from build123d import *

# Parameters (mm, degrees)
F1_DEPTH     = 1016
F2_R         = 25.4
F3_T1_DEPTH  = 1143
F3_T4_ANGLE  = 90
F3_T6_ANGLE  = 90
F3_T8_ANGLE  = 90
F3_T10_ANGLE = 90
F4_T         = -2.54


# Not quite as in the source:
# - a fillet or chamfer that OpenCascade refuses, or shapes differently, is made with other operations: its cross-section is extruded or revolved along the edge and cut away or added


with BuildPart() as f1:
    # F0 (on Top) → F1 (new body)
    with BuildSketch(Plane.XY):
        Polygon((254, -254), (254, 0), (254, 254), (-254, 254), (-254, -254), align=None)
    extrude(amount=F1_DEPTH)

    # F2
    f2_edges = [f1.edges().sort_by_distance(p)[0] for p in [
        (-254, 0, 0),
        (0, 254, 0),
        (0, -254, 0),
        (254, 0, 0),
    ]]
    fillet(f2_edges, radius=F2_R)

    # F3: fillet of radius 50.8 on 4 edges, made by hand

    # F3_s2 → F3_t1 (cut)
    with BuildSketch(Plane.XY):
        with BuildLine():
            ThreePointArc((-203.2, 254), (-239.1210244843, 239.1210244843), (-254, 203.2))
            Line((-254, 203.2), (-254, 254))
            Line((-254, 254), (-203.2, 254))
        make_face()
        with BuildLine():
            ThreePointArc((-203.2, -254), (-239.1210244843, -239.1210244843), (-254, -203.2))
            Line((-254, -203.2), (-254, -254))
            Line((-254, -254), (-203.2, -254))
        make_face()
        with BuildLine():
            ThreePointArc((254, 203.2), (239.1210244843, 239.1210244843), (203.2, 254))
            Line((203.2, 254), (254, 254))
            Line((254, 254), (254, 203.2))
        make_face()
        with BuildLine():
            ThreePointArc((254, -203.2), (239.1210244843, -239.1210244843), (203.2, -254))
            Line((203.2, -254), (254, -254))
            Line((254, -254), (254, -203.2))
        make_face()
    extrude(amount=F3_T1_DEPTH, mode=Mode.SUBTRACT)

    # F3_s3 → F3_t4 (revolve, cut)
    with BuildSketch(Plane.XZ.offset(203.2)):
        with BuildLine():
            ThreePointArc((228.6, 0), (246.5605122421, 7.4394877579), (254, 25.4))
            Line((254, 25.4), (254, 0))
            Line((254, 0), (228.6, 0))
        make_face()
    revolve(axis=Axis((203.2, -203.2, 0), (0, 0, -1)), revolution_arc=F3_T4_ANGLE, mode=Mode.SUBTRACT)

    # F3_s5 → F3_t6 (revolve, cut)
    with BuildSketch(Plane.YZ.offset(203.2)):
        with BuildLine():
            ThreePointArc((228.6, 0), (246.5605122421, 7.4394877579), (254, 25.4))
            Line((254, 25.4), (254, 0))
            Line((254, 0), (228.6, 0))
        make_face()
    revolve(axis=Axis((203.2, 203.2, 0), (0, 0, -1)), revolution_arc=F3_T6_ANGLE, mode=Mode.SUBTRACT)

    # F3_s7 → F3_t8 (revolve, cut)
    with BuildSketch(Plane.YZ.offset(-203.2)):
        with BuildLine():
            ThreePointArc((-228.6, 0), (-246.5605122421, 7.4394877579), (-254, 25.4))
            Line((-254, 25.4), (-254, 0))
            Line((-254, 0), (-228.6, 0))
        make_face()
    revolve(axis=Axis((-203.2, -203.2, 0), (0, 0, -1)), revolution_arc=F3_T8_ANGLE, mode=Mode.SUBTRACT)

    # F3_s9 → F3_t10 (revolve, cut)
    with BuildSketch(Plane.XZ.offset(-203.2)):
        with BuildLine():
            ThreePointArc((-228.6, 0), (-246.5605122421, 7.4394877579), (-254, 25.4))
            Line((-254, 25.4), (-254, 0))
            Line((-254, 0), (-228.6, 0))
        make_face()
    revolve(axis=Axis((-203.2, 203.2, 0), (0, 0, -1)), revolution_arc=F3_T10_ANGLE, mode=Mode.SUBTRACT)

    # F4
    f4_openings = [f1.faces().sort_by_distance(p)[0] for p in [
        (0, 0, 1016),
    ]]
    offset(amount=F4_T, openings=f4_openings)


solid = f1.part
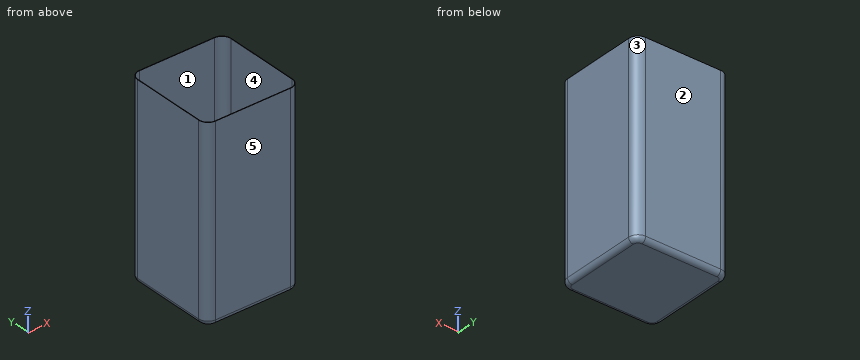
Design review of the part built by this model. Coordinates are the model's own, in mm. Face numbers are marked on the shaded views. A direction names the side the tool comes from. Coordinates: 2 decimals unless noted, no trailing zeros. Order: outer loops, then holes, each group sorted by start corner. A loop starts at its lowest first (then second) coordinate and runs counter-clockwise, first axis right, second up.
Item 1: The part is to be moulded in two halves that separate along X. For the marked faces 3, 4 and 5, say which applies: pulls with the +X half, pulls with the -X half, needs draft (parallel to the pull), parting line crosses it, or undercut.
Item 2: For pin 1 Ø1 at (x, y) = (34.5, -71.5) entering from +Z, flat-tipped, find the tip position at first contact; note if it passes through.
Item 3: Take a section at B-B, the plane x = 115.5. Write out the cut boundary in (y, z), then the cut area to 3 significant figures.
Item 4: For line 1 (X direction, y = -106, z = 292); line 2 (Z direction, x = -77, y = 9.5), list the stretches that pass through material, from the lowest coordinate up.
Item 5: For the marked faces 1 and 2, list the 3-axis set-ups (+Z, -Z, +X, -X, +Y, -Y) from which the entire face can be reached by the end or side of a thin tool; tool diameter is ignored.
Item 6: Take a section at A-A, the plane z = 389. Write out the cut boundary in (x, y).
The answers:
1. face 3: pulls with the +X half
1. face 4: undercut
1. face 5: needs draft
2. pin 1: stops at z = 2.54
3. outline: (-254, 25.4) arc R25.4 ccw to (-228.6, 0) - (228.6, 0) arc R25.4 ccw to (254, 25.4) - (254, 1016) - (251.46, 1016) - (251.46, 25.4) arc R22.86 cw to (228.6, 2.54) - (-228.6, 2.54) arc R22.86 cw to (-251.46, 25.4) - (-251.46, 1016) - (-254, 1016) - close
3. area: 6,390 mm2
4. line 1: x = -254 to -251.46, 251.46 to 254
4. line 2: z = 0 to 2.54
5. face 1: +Z
5. face 2: +Z, -Z, +X, -X, +Y
6. outline: (-254, -203.2) arc R50.8 ccw to (-203.2, -254) - (203.2, -254) arc R50.8 ccw to (254, -203.2) - (254, 203.2) arc R50.8 ccw to (203.2, 254) - (-203.2, 254) arc R50.8 ccw to (-254, 203.2) - close; hole (-251.46, -203.2) arc R48.26 ccw to (-203.2, -251.46) - (203.2, -251.46) arc R48.26 ccw to (251.46, -203.2) - (251.46, 203.2) arc R48.26 ccw to (203.2, 251.46) - (-203.2, 251.46) arc R48.26 ccw to (-251.46, 203.2) - close
